from build123d import *

# Parameters (mm, degrees)
F0_W          = 55.6310900272
F0_H          = 20
F1_DEPTH      = 8
F2_W          = 2.5
F2_H          = 40
F3_DEPTH      = 27.8165450136
F3_DEPTH_BACK = 25
F5_DEPTH      = 10


# Not quite as in the source:
# - a feature names something its author has since deleted; it is built from what else it names


with BuildPart() as f1:
    # F0 (on Front) → F1 (new body)
    with BuildSketch(Plane.XZ):
        Rectangle(F0_W, F0_H)
    extrude(amount=-F1_DEPTH)

    # F2 (on Right) → F3 (cut, two sides)
    with BuildSketch(Plane.YZ) as f3_sk:
        with Locations((3.9288233686, 0)):
            Rectangle(F2_W, F2_H)
    extrude(amount=F3_DEPTH, mode=Mode.SUBTRACT)
    extrude(f3_sk.sketch, amount=-F3_DEPTH_BACK, mode=Mode.SUBTRACT)

    # F4 (on Top) → F5 (join, symmetric)
    with BuildSketch(Plane.XY):
        Polygon((24.1118337571, 28.2883709489), (-27.8155450136, 14.3744717422), (-27.8155450136, 8), (-24.8155450136, 8), (-24.8155450136, 12.0724907783), (24.1118337571, 25.1825424077), align=None)
        Polygon((27.1118309825, 28.2842907635), (24.1118337571, 28.2883709489), (24.1118337571, 25.1825424077), (24.1118337571, 22.2315117717), (27.1118309825, 22.2315117717), align=None)
    extrude(amount=F5_DEPTH, both=True)


solid = f1.part
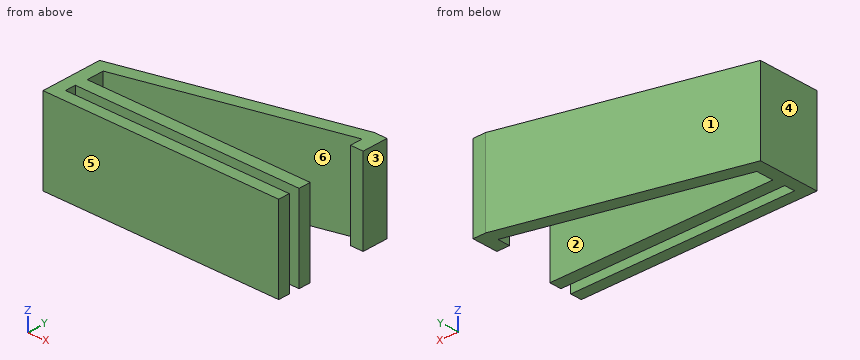
Verification items for the finished model (mm, model axes). Face numbers are marked on the shaded views. A direction names the side the tool comes from. Round coordinates to 2 decimals unless told otherwise and drop trailing zeros. Loops run counter-clockwise (first coordinate to the right, second up) from the corner with the lowest first, then second, coordinate; pieces in that order, holes last. Notation, with made-up numbers: (-35, -4.5) - (5, -4.5) arc R16 cw to (5, 20.5) - close; hole circle Ø3 at (76.5, 31). An arc over 180 degrees is marked (long way). Use one line per item in the form item = value.
1. Section check A-A on y = 24.5. Record the cut outline in (x, z).
A:
outline = (9.97, -10) - (21.56, -10) - (21.56, 10) - (9.97, 10) - close; (24.11, -10) - (27.11, -10) - (27.11, 10) - (24.11, 10) - close
2. Gauge pin test, flat ends, axial feed: pin 1 Ø10 at (x, z) = (-8.5, -5) entering from +Y; pin 2 Ø4 at (y, z) = (21.5, -5.5) entering from +X; pin 3 Ø1 at (x, z) = (-11, 0.5) entering from +Y. Record the tip position at first contact, or that the pin passes through.
A:
pin_1 = 20.89
pin_2 = 27.11
pin_3 = 19.01
3. Scan lines: probe 1 along Y at (x, z) = (26.5, 6.5); probe 2 along Y at (x, z) = (22, 2.5); probe 3 along X at (y, z) = (10, -0.5). Record each from-to range of solid material in increasing order.
A:
probe_1 = 0 to 2.68, 5.18 to 8, 22.23 to 28.29
probe_2 = 0 to 2.68, 5.18 to 8, 24.62 to 27.72
probe_3 = -27.82 to -24.82
4. Access from +Z, -Z, +X, -X, +Y, -Y to the whole of each face (thin tool, end or side, straight path). Record for the marked faces 1, 2 and 3.
A:
face_1 = +Z, -Z, -X, +Y
face_2 = +Z, -Z, +X
face_3 = +Z, -Z, +X, +Y
5. Section check D-D on y = 3.5. Record the cut outline in (x, z), and give its area (3 significant figures).
A:
outline = (-27.82, -10) - (-25, -10) - (-25, 10) - (-27.82, 10) - close
area = 56.3 mm²
6. Section check C-C on x = 17.5. Record the cut outline in (y, z), and give its area (3 significant figures).
A:
outline = (0, -10) - (2.68, -10) - (2.68, 10) - (0, 10) - close; (5.18, -10) - (8, -10) - (8, 10) - (5.18, 10) - close; (23.41, -10) - (26.52, -10) - (26.52, 10) - (23.41, 10) - close
area = 172 mm²
7. Section check B-B on z = -2.5. Record the cut outline in (x, y), and give its area (3 significant figures).
A:
outline = (-27.82, 0) - (27.82, 0) - (27.82, 2.68) - (-25, 2.68) - (-25, 5.18) - (27.82, 5.18) - (27.82, 8) - (-24.82, 8) - (-24.82, 12.07) - (24.11, 25.18) - (24.11, 22.23) - (27.11, 22.23) - (27.11, 28.28) - (24.11, 28.29) - (-27.82, 14.37) - close
area = 503 mm²
8. Draft check along Y on the marked faces 4, 5 and 6. Enter one of: pulls with the +Y half, pulls with the -Y half, needs draft (parallel to the pull), parting line crosses it, or undercut.
A:
face_4 = needs draft
face_5 = pulls with the -Y half
face_6 = undercut
